```python
from build123d import *

# Parameters (mm, degrees)
SKETCH_1_W          = 65
SKETCH_1_H          = 55
SKETCH_1_W_2        = 55
SKETCH_1_H_2        = 45
EXTRUDE_1_DEPTH     = 90
SKETCH_2_W          = 65
SKETCH_2_H          = 55
EXTRUDE_2_DEPTH     = 4
SKETCH_3_W          = 65
SKETCH_3_H          = 15
EXTRUDE_3_DEPTH     = 5
EXTRUDE_4_DEPTH     = 5
EXTRUDE_5_DEPTH     = 5
SKETCH_6_R          = 1.6
CUT_EXTRUDE_1_DEPTH = 124.895116934
SKETCH_7_R          = 1.6
EXTRUDE_6_DEPTH     = 5
SKETCH_8_R          = 1.6
EXTRUDE_7_DEPTH     = 5
EXTRUDE_START       = 8
SKETCH_9_R          = 7.5
SKETCH_9_R_2        = 1.6
EXTRUDE_9_DEPTH     = 8
SKETCH_10_W         = 49
SKETCH_10_H         = 51.68
CUT_EXTRUDE_2_DEPTH = 130.421791055
SKETCH_12_W         = 37
SKETCH_12_H         = 37
CUT_EXTRUDE_3_DEPTH = 134.018795664
FILLET_2_R          = 8
FILLET_3_R          = 5


with BuildPart() as part:
    # 草图1 → 凸台-拉伸1 (new body)
    with BuildSketch(Plane(origin=(0, 0, 0), x_dir=(1, 0, 0), z_dir=(0, 1, 0))):
        with Locations((32.5, 27.5)):
            Rectangle(SKETCH_1_W, SKETCH_1_H)
        with Locations((32.5, 27.5)):
            Rectangle(SKETCH_1_W_2, SKETCH_1_H_2, mode=Mode.SUBTRACT)
    extrude(amount=EXTRUDE_1_DEPTH)

    # 草图2 → 凸台-拉伸2 (add)
    with BuildSketch(Plane.XZ):
        with Locations((32.5, -27.5)):
            Rectangle(SKETCH_2_W, SKETCH_2_H)
    extrude(amount=EXTRUDE_2_DEPTH)

    # 草图3 → 凸台-拉伸3 (add)
    with BuildSketch(Plane(origin=(0, 0, -55), x_dir=(-1, 0, 0), z_dir=(0, 0, -1))):
        with Locations((-32.5, -11.5)):
            Rectangle(SKETCH_3_W, SKETCH_3_H)
    extrude(amount=-EXTRUDE_3_DEPTH)

    # 草图4 → 凸台-拉伸4 (add)
    with BuildSketch(Plane(origin=(65, 0, 0), x_dir=(0, 0, -1), z_dir=(1, 0, 0))):
        Polygon((0, -4), (50, -19), (50, -4), align=None)
    extrude(amount=-EXTRUDE_4_DEPTH)

    # 草图5 → 凸台-拉伸5 (add)
    with BuildSketch(Plane.ZY):
        Polygon((-50, -19), (0, -4), (-50, -4), align=None)
    extrude(amount=-EXTRUDE_5_DEPTH)

    # 草图6 → 切除-拉伸1 (cut, through all)
    with BuildSketch(Plane(origin=(0, 0, -55), x_dir=(-1, 0, 0), z_dir=(0, 0, -1))):
        with Locations((-12.5, -11.5)):
            Circle(SKETCH_6_R)
        with Locations((-52.5, -11.5)):
            Circle(SKETCH_6_R)
    extrude(amount=-CUT_EXTRUDE_1_DEPTH, mode=Mode.SUBTRACT)

    # 草图7 → 凸台-拉伸6 (add)
    # profile 1 of 2: a face of its own
    with BuildSketch(Plane(origin=(0, 0, -55), x_dir=(-1, 0, 0), z_dir=(0, 0, -1))):
        with BuildLine():
            Line((0, 78.68), (0, 58.68))
            ThreePointArc((0, 58.68), (1.464466094, 62.215533906), (5, 63.68))
            ThreePointArc((5, 63.68), (10, 68.68), (5, 73.68))
            ThreePointArc((5, 73.68), (1.464466094, 75.144466094), (0, 78.68))
        make_face()
        with Locations((5, 68.68)):
            Circle(SKETCH_7_R, mode=Mode.SUBTRACT)
    # profile 2 of 2: a face of its own
    with BuildSketch(Plane(origin=(0, 0, -55), x_dir=(-1, 0, 0), z_dir=(0, 0, -1))):
        with BuildLine():
            Line((-65, 78.68), (-65, 58.68))
            ThreePointArc((-65, 58.68), (-66.464466094, 62.215533906), (-70, 63.68))
            ThreePointArc((-70, 63.68), (-75, 68.68), (-70, 73.68))
            ThreePointArc((-70, 73.68), (-66.464466094, 75.144466094), (-65, 78.68))
        make_face()
        with Locations(Location((-70, 68.68, 0), (0, 0, 180))):
            Circle(SKETCH_7_R, mode=Mode.SUBTRACT)
    extrude(amount=-EXTRUDE_6_DEPTH)

    # 草图8 → 凸台-拉伸7 (add)
    # profile 1 of 3: a face of its own
    with BuildSketch(Plane.XY):
        with BuildLine():
            Line((71.150434847, 88.545850354), (65, 90))
            Line((65, 90), (65, 73.68))
            ThreePointArc((65, 73.68), (66.464466094, 77.215533906), (70, 78.68))
            ThreePointArc((70, 78.68), (74.966349352, 83.100885058), (71.150434847, 88.545850354))
        make_face()
        with Locations((70, 83.68)):
            Circle(SKETCH_8_R, mode=Mode.SUBTRACT)
    # profile 2 of 3: a face of its own
    with BuildSketch(Plane.XY):
        with BuildLine():
            Line((0, 90), (0, 73.68))
            ThreePointArc((0, 73.68), (-1.464466094, 77.215533906), (-5, 78.68))
            ThreePointArc((-5, 78.68), (-9.966349352, 83.100885058), (-6.150434847, 88.545850354))
            Line((-6.150434847, 88.545850354), (0, 90))
        make_face()
        with Locations(Location((-5, 83.68, 0), (0, 0, 180))):
            Circle(SKETCH_8_R, mode=Mode.SUBTRACT)
    # profile 3 of 3: a face of its own
    with BuildSketch(Plane.XY):
        with BuildLine():
            Line((42.5, -4), (22.5, -4))
            ThreePointArc((22.5, -4), (26.035533906, -5.464466094), (27.5, -9))
            ThreePointArc((27.5, -9), (32.5, -14), (37.5, -9))
            ThreePointArc((37.5, -9), (38.964466094, -5.464466094), (42.5, -4))
        make_face()
        with Locations((32.5, -9)):
            Circle(SKETCH_8_R, mode=Mode.SUBTRACT)
    extrude(amount=-EXTRUDE_7_DEPTH)

    # 草图9 → 凸台-拉伸9 (add)
    # profile 1 of 3: a face of its own
    with BuildSketch(Plane(origin=(0, 0, -55), x_dir=(-1, 0, 0), z_dir=(0, 0, -1)).offset(EXTRUDE_START)):
        with Locations(Location((-52.5, -11.5, 0), (0, 0, 270))):
            Circle(SKETCH_9_R)
        with Locations((-52.5, -11.5)):
            Circle(SKETCH_9_R_2, mode=Mode.SUBTRACT)
    # profile 2 of 3: a face of its own
    with BuildSketch(Plane(origin=(0, 0, -55), x_dir=(-1, 0, 0), z_dir=(0, 0, -1)).offset(EXTRUDE_START)):
        with Locations(Location((-12.5, -11.5, 0), (0, 0, 270))):
            Circle(SKETCH_9_R)
        with Locations((-12.5, -11.5)):
            Circle(SKETCH_9_R_2, mode=Mode.SUBTRACT)
    # profile 3 of 3: a face of its own
    with BuildSketch(Plane(origin=(0, 0, -55), x_dir=(-1, 0, 0), z_dir=(0, 0, -1)).offset(EXTRUDE_START)):
        with BuildLine():
            Line((-70, 73.68), (5, 73.68))
            ThreePointArc((5, 73.68), (10, 68.68), (5, 63.68))
            Line((5, 63.68), (-70, 63.68))
            ThreePointArc((-70, 63.68), (-75, 68.68), (-70, 73.68))
        make_face()
        with Locations((5, 68.68)):
            Circle(SKETCH_9_R_2, mode=Mode.SUBTRACT)
        with Locations((-70, 68.68)):
            Circle(SKETCH_9_R_2, mode=Mode.SUBTRACT)
    extrude(amount=-EXTRUDE_9_DEPTH)

    # 草图10 → 切除-拉伸2 (cut, through all)
    with BuildSketch(Plane(origin=(0, 0, -55), x_dir=(-1, 0, 0), z_dir=(0, 0, -1))):
        with Locations((-32.5, 29.84)):
            Rectangle(SKETCH_10_W, SKETCH_10_H)
    extrude(amount=-CUT_EXTRUDE_2_DEPTH, mode=Mode.SUBTRACT)

    # 草图12 → 切除-拉伸3 (cut, through all)
    with BuildSketch(Plane.ZY):
        with Locations((-27.5, 67.5)):
            Rectangle(SKETCH_12_W, SKETCH_12_H)
        with Locations((-27.5, 22.5)):
            Rectangle(SKETCH_12_W, SKETCH_12_H)
    extrude(amount=-CUT_EXTRUDE_3_DEPTH, mode=Mode.SUBTRACT)

    # 圆角2
    fillet_2_edges = [part.edges().sort_by_distance(p)[0] for p in [
        (62.5, 4, -46),
        (2.5, 4, -46),
        (62.5, 4, -9),
        (2.5, 4, -9),
        (62.5, 86, -46),
        (2.5, 86, -46),
        (62.5, 86, -9),
        (2.5, 86, -9),
    ]]
    fillet(fillet_2_edges, radius=FILLET_2_R)

    # 圆角3
    fillet_3_edges = [part.edges().sort_by_distance(p)[0] for p in [
        (57, 55.68, -2.5),
        (8, 55.68, -2.5),
        (8, 4, -2.5),
        (57, 4, -2.5),
        (57, 55.68, -52.5),
        (8, 55.68, -52.5),
        (8, 4, -52.5),
        (57, 4, -52.5),
    ]]
    fillet(fillet_3_edges, radius=FILLET_3_R)


solid = part.part
```
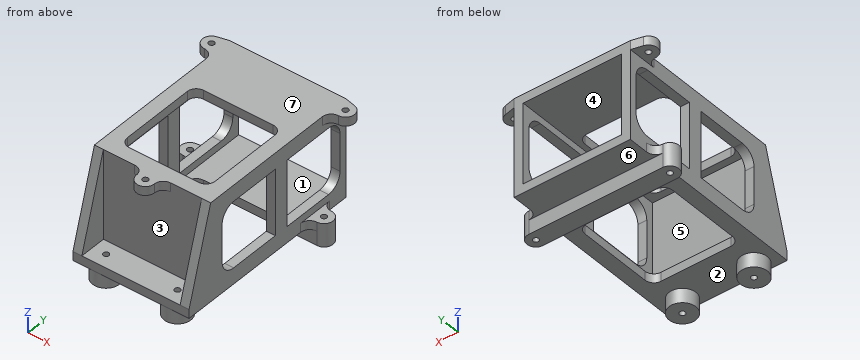
Geometry: final body of the model. Coordinates: model frame, mm. Face numbers are marked on the shaded views. A direction names the side the tool comes from. Coordinates: 2 decimals unless noted, no trailing zeros. Order: outer loops, then holes, each group sorted by start corner. A loop starts at its lowest first (then second) coordinate and runs counter-clockwise, first axis right, second up.
Item 1: Section query A-A (z = -34.5). Output: boundary loops of the cut face in (x, y).
Answer:
outline: (0, -14.35) - (5, -14.35) - (5, -4) - (60, -4) - (60, -14.35) - (65, -14.35) - (65, 4) - (60, 4) - (60, 0) - (5, 0) - (5, 4) - (0, 4) - close; (0, 41) - (5, 41) - (5, 49) - (0, 49) - close; (0, 86) - (5, 86) - (5, 90) - (0, 90) - close; (60, 41) - (65, 41) - (65, 49) - (60, 49) - close; (60, 86) - (65, 86) - (65, 90) - (60, 90) - close
Item 2: Material intervals for line 1 along X through (y, z) = (83.68, -2.45); line 2 along X through (y, z) = (-11, -60); line 3 along Z through (x, y) = (57.5, 4), sorted ascending.
Answer:
line 1: x = -10 to -6.6, -3.4 to 68.4, 71.6 to 75
line 2: x = 5.02 to 10.98, 14.02 to 19.98, 45.02 to 50.98, 54.02 to 59.98
line 3: z = -55 to -50, -5 to 0
Item 3: Access query for the marked faces 1, 2 and 3. Directions: +Z, -Z, +X, -X, +Y, -Y. A direction counts if a zero-diameter tool reaches every point of the face in a straight line with its end or side. Return the directions, or none.
Answer:
face 1: +Y
face 2: -Z
face 3: -Y
Item 4: Section query C-C (x = 63.5). Output: boundary loops of the cut face in (y, z).
Answer:
outline: (-19, -55) - (63.68, -55) - (63.68, -63) - (73.68, -63) - (73.68, -55) - (90, -55) - (90, 0) - (-4, 0) - (-19, -50) - close; hole (4, -38) arc R8 ccw to (12, -46) - (41, -46) - (41, -9) - (12, -9) arc R8 ccw to (4, -17) - close; hole (49, -46) - (78, -46) arc R8 ccw to (86, -38) - (86, -17) arc R8 ccw to (78, -9) - (49, -9) - close
Item 5: Draft query along Z for the marked faces 4, 5, 6 and 7. Return one class per face: released by +Z, released by -Z, zero draft, split by the parting line, or undercut.
Answer:
face 4: undercut
face 5: undercut
face 6: released by -Z
face 7: released by +Z
Item 6: Contact query for flat-ended pins moving along their axis: P1, Ø8, axis at y = 68, z = -14.5, coming from the +X side; P2, Ø6, axis at y = 62, z = -45, coming from the -X side; P3, Ø2, axis at x = 52.5, y = -1.5, coming from the -Z side; P4, Ø3.5, axis at x = 12.5, y = -11.5, coming from the +Z side. Output: stop coordinate, or through.
Answer:
P1: passes through
P2: stops at x = 0
P3: stops at z = -55
P4: stops at z = -50
Item 7: Section query B-B (x = 25.5). Output: boundary loops of the cut face in (y, z).
Answer:
outline: (-19, -55) - (4, -55) - (4, -50) - (0, -50) - (0, -5) - (4, -5) - (4, 0) - (-5, 0) - (-5, -5) - (-4, -5) - (-4, -50) - (-19, -50) - close; (55.68, -55) - (63.68, -55) - (63.68, -63) - (73.68, -63) - (73.68, -55) - (90, -55) - (90, -50) - (55.68, -50) - close; (55.68, -5) - (90, -5) - (90, 0) - (55.68, 0) - close
Item 8: Section query D-D (y = 83.68). Output: boundary loops of the cut face in (x, z), then the cut area to 3 significant figures.
Answer:
outline: (-10, -5) - (-6.6, -5) - (-6.6, 0) - (-10, 0) - close; (-3.4, -5) - (0, -5) - (0, -11.37) - (5, -11.37) - (5, -5) - (60, -5) - (60, -11.37) - (65, -11.37) - (65, -5) - (68.4, -5) - (68.4, 0) - (-3.4, 0) - close; (0, -55) - (65, -55) - (65, -43.63) - (60, -43.63) - (60, -50) - (5, -50) - (5, -43.63) - (0, -43.63) - close; (71.6, -5) - (75, -5) - (75, 0) - (71.6, 0) - close
area: 845 mm2
